Verification items for the finished model (mm, model axes). A direction names the side the tool comes from. Give positions to 0.01 mm unless a question says otherwise; leave off trailing zeros. Write each loop counter-clockwise with the first axis right and the second up, starting at its lowest first coordinate (ties: lowest second). Pieces come first, ordered by that corner, then holes. Notation, with made-up numbers: (3.5, -24) -> (43.5, -24) arc R28 cw to (43.5, -2) -> close; hole circle Ø9 at (6.25, 26.5). An arc over 180 degrees is marked (long way). Write item = value, one per line.
from build123d import *
from OCP.BRepFilletAPI import BRepFilletAPI_MakeChamfer

# Parameters (mm, degrees)
SKETCH1_R           = 1.0668
BOSS_EXTRUDE1_DEPTH = 7.5
BOSS_EXTRUDE2_DEPTH = 7.8
BOSS_EXTRUDE3_START = 7.7
SKETCH3_R           = 1.0668
BOSS_EXTRUDE3_DEPTH = 7.7
BOSS_EXTRUDE4_DEPTH = 23
CHAMFER1_SIZE       = 2.6
CHAMFER1_SIZE2      = 5.575717993


with BuildPart() as part:
    # Sketch1 → Boss-Extrude1 (new body)
    with BuildSketch(Plane.XY):
        with BuildLine():
            Line((0, 0), (6.519373857, 0.102105999))
            add(Edge.make_bspline(
                [(6.519373857, 0.102105999), (7.62, 0.119343933), (8.701246874, 0.325693755)],
                knots=[0, 0, 0, 1, 1, 1], degree=2))
            Line((8.701246874, 0.325693755), (14.703179453, 1.471128487))
            ThreePointArc((14.703179453, 1.471128487), (16.587758943, 4.427434521), (13.526155588, 6.135641216))
            add(Edge.make_bspline(
                [(13.526155588, 6.135641216), (12.7, 5.874844246), (12.7, 6.741186046)],
                knots=[0, 0, 0, 1, 1, 1], degree=2))
            Line((12.7, 6.741186046), (12.7, 9.241186046))
            Line((12.7, 9.241186046), (-4.709853694, 0))
            Line((-4.709853694, 0), (0, 0))
        make_face()
        with Locations((12.7, 3.481838658)):
            Circle(SKETCH1_R, mode=Mode.SUBTRACT)
        with Locations((7.617577591, 2.105666766)):
            Circle(SKETCH1_R, mode=Mode.SUBTRACT)
    extrude(amount=BOSS_EXTRUDE1_DEPTH)

    # Sketch2 → Boss-Extrude2 (add)
    with BuildSketch(Plane(origin=(0, 0, 0), x_dir=(-1, 0, 0), z_dir=(0, 0, -1))):
        Polygon((-12.7, 6.741186046), (4.709853694, 0), (-12.7, 9.241186046), align=None)
    extrude(amount=BOSS_EXTRUDE2_DEPTH)

    # Sketch3 → Boss-Extrude3 (add)
    with BuildSketch(Plane(origin=(0, 0, -7.8), x_dir=(-1, 0, 0), z_dir=(0, 0, -1)).offset(BOSS_EXTRUDE3_START)):
        with BuildLine():
            Line((-12.7, 9.241186046), (-12.7, 6.741186047))
            add(Edge.make_bspline(
                [(-12.7, 6.741186047), (-12.7, 5.874844247), (-13.526155587, 6.135641216)],
                knots=[0, 0, 0, 1, 1, 1], degree=2))
            ThreePointArc((-13.526155587, 6.135641216), (-16.587758943, 4.427434521), (-14.703179453, 1.471128487))
            Line((-14.703179453, 1.471128487), (-8.70124687, 0.325693755))
            add(Edge.make_bspline(
                [(-8.70124687, 0.325693755), (-7.619999998, 0.119343933), (-6.519373857, 0.102105999)],
                knots=[0, 0, 0, 1, 1, 1], degree=2))
            Line((-6.519373857, 0.102105999), (0, 0))
            Line((0, 0), (4.709853694, 0))
            Line((4.709853694, 0), (-12.7, 9.241186046))
        make_face()
        with Locations(Location((-12.7, 3.481838658, 0), (0, 0, 180))):
            Circle(SKETCH3_R, mode=Mode.SUBTRACT)
        with Locations(Location((-7.617577591, 2.105666766, 0), (0, 0, 180))):
            Circle(SKETCH3_R, mode=Mode.SUBTRACT)
    extrude(amount=-BOSS_EXTRUDE3_DEPTH)

    # Sketch4 → Boss-Extrude4 (add)
    with BuildSketch(Plane.XY.offset(7.5)):
        with BuildLine():
            Line((0, 0), (4.638040447, 0.072640681))
            ThreePointArc((4.638040447, 0.072640681), (2.936201023, 1.452503315), (3.995073153, 3.370593023))
            Line((3.995073153, 3.370593023), (3.995073153, 4.620593023))
            Line((3.995073153, 4.620593023), (-4.709853694, 0))
            Line((-4.709853694, 0), (0, 0))
        make_face()
    extrude(amount=-BOSS_EXTRUDE4_DEPTH)

    # Chamfer1: one chamfer whose edges measure the first distance from different faces: ONE call of the kernel's chamfer builder (chamfer() names one face for all edges)
    chamfer1_edges_1 = [part.edges().sort_by_distance(p)[0] for p in [
        (3.995073153, 4.620593023, 7.5),
    ]]
    chamfer1_side_1 = [part.faces().sort_by_distance(p)[0] for p in [
        (7.962373857, 3.352750827, 7.5),
    ]]
    chamfer1_edges_2 = [part.edges().sort_by_distance(p)[0] for p in [
        (3.995073153, 4.620593023, -15.5),
    ]]
    chamfer1_side_2 = [part.faces().sort_by_distance(p)[0] for p in [
        (7.962373857, 3.352750827, -15.5),
    ]]
    chamfer1 = BRepFilletAPI_MakeChamfer(part.part.solid().wrapped)
    for e in chamfer1_edges_1:
        chamfer1.Add(CHAMFER1_SIZE, CHAMFER1_SIZE2, e.wrapped, chamfer1_side_1[0].wrapped)  # the first distance lies on this face
    for e in chamfer1_edges_2:
        chamfer1.Add(CHAMFER1_SIZE, CHAMFER1_SIZE2, e.wrapped, chamfer1_side_2[0].wrapped)  # the first distance lies on this face
    add(Compound.cast(chamfer1.Shape()), mode=Mode.REPLACE)


solid = part.part
Item 1: Sectioned sample at D-D on y = 5.25. Record the cut outline in (x, z), then the cut area to 3 significant figures.
Response values:
outline = (5.18, -9.92) -> (10.73, -15.5) -> (16.2, -15.5) -> (16.2, -7.8) -> (8.85, -7.8) -> (8.85, 0) -> (16.2, 0) -> (16.2, 7.5) -> (10.73, 7.5) -> (5.18, 1.92) -> close
area = 165 mm^2
Item 2: Material ranges on line 1 (Z direction, x = 9, y = 1.5); line 2 (X direction, y = 2.75, z = 4); line 3 (Z direction, x = 4.25, y = 2.5), recorded low to high.
Response values:
line_1 = -15.5 to -7.8, 0 to 7.5
line_2 = 2.54 to 6.77, 8.47 to 11.92, 13.48 to 16.4
line_3 = -14.2 to -7.8, 0 to 6.2
Item 3: Sectioned sample at B-B on y = 4. Record the cut outline in (x, z), then the cut area to 3 significant figures.
Response values:
outline = (2.83, -9.92) -> (8.37, -15.5) -> (11.77, -15.5) -> (11.77, -7.8) -> (5.62, -7.8) -> (5.62, 0) -> (11.77, 0) -> (11.77, 7.5) -> (8.37, 7.5) -> (2.83, 1.92) -> close; (13.63, -15.5) -> (16.66, -15.5) -> (16.66, -7.8) -> (13.63, -7.8) -> close; (13.63, 0) -> (16.66, 0) -> (16.66, 7.5) -> (13.63, 7.5) -> close
area = 173 mm^2
Item 4: Set-up check for faces 4 (the flat face through (3.873, 4.556, -4.083)), 5 (the flat face through (12.7, 8, -4)): record each of +Z, -Z, +X, -X, +Y, -Y from which the full face is reachable in a straight line by a thin tool's end or side.
Response values:
face_4 = +Z, -Z, -X, +Y
face_5 = +Z, -Z, +X, +Y
Item 5: Sectioned sample at A-A on x = 3.25. Record the cut outline in (y, z).
Response values:
outline = (0.05, -15.5) -> (1.28, -15.5) -> (4.23, -9.92) -> (4.23, 1.92) -> (1.28, 7.5) -> (0.05, 7.5) -> close; hole (0.75, -7.8) -> (2.81, -7.8) -> (2.81, 0) -> (0.75, 0) -> close
Item 6: Mould release check, pull along Z, two halves, no side actions. Record for faces 1 (the flat face through (8.41, 5.08, -3.85)), 2 (the flat face through (11.7, 0.9, 3.7)), 3 (the flat face through (10, 3, 7.5)): +Z half, -Z half, draft (parallel to the pull), parting line (faces both ways), or undercut.
Response values:
face_1 = undercut
face_2 = draft
face_3 = +Z half
Item 7: Sectioned sample at C-C on z = -1.25. Record the cut outline in (x, y).
Response values:
outline = (-4.71, 0) -> (0, 0) -> (4.64, 0.07) arc R1.71 cw to (4, 3.37) -> (12.7, 6.74) -> (12.7, 9.24) -> close
Item 8: Go/stop test with flat-tipped pins: P1, Ø3, axis at y = 7.5, z = -2.5, coming from the +X side; P2, Ø6, axis at x = 10, z = -9, coming from the -Y side; P3, Ø6, axis at x = 0.5, z = 3, coming from the +Y side; P4, Ø1.5, axis at x = 3, y = 7, coming from the -Z side. Record where each tip stops, or that it passes through.
Response values:
P1 = 12.7
P2 = 0.12
P3 = 4.25
P4 = through
